For this review, use the dimensioned drawing (mm, ordinates from the lowest corner) and the shaded views. Coordinates: 2 decimals unless noted, no trailing zeros. Write each loop counter-clockwise with the first axis right and the second up, starting at its lowest first coordinate (ties: lowest second). Pieces come first, ordered by that corner, then holes. Notation, with made-up numbers: (-34, 5.5) - (-6, 5.5) arc R15 cw to (-6, 26.5) - close; hole circle Ø5 at (77.5, 70.25). An arc over 180 degrees is marked (long way). One line per item, written item: value.
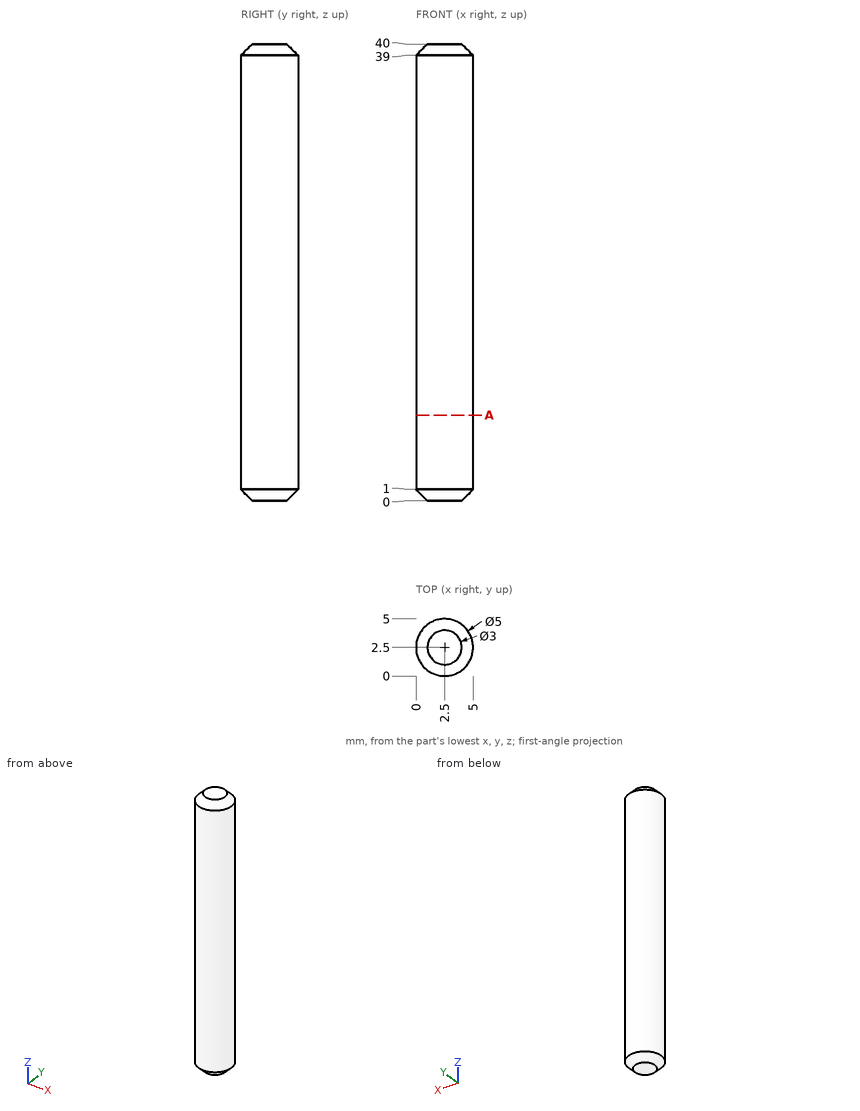
1. Consider section A-A, the plane z = 7.5. Write out the cut boundary in (x, y), then the cut area to 3 significant figures.
Answer block:
outline: circle Ø5 at (2.5, 2.5)
area: 19.6 mm^2
2. Wall thickness on line 1 along Y through (x, z) = (0.5, 24.5); line 2 along Y through (x, z) = (2.35, 15); line 3 along X through (y, z) = (0.95, 7.5): over which ranges is each line inside the solid? List them lowest first.
Answer block:
line 1: y = 1 to 4
line 2: y = 0 to 5
line 3: x = 0.54 to 4.46
3. Insertion check: pin 1 Ø1 at (y, z) = (4.5, 12) entering from +X. The pin has a flat end and moves straight along its axis. Give the tip position at first contact, or say it passes through.
Answer block:
pin 1: stops at x = 4.5
